```python
from build123d import *

# Parameters (mm, degrees)
F0_R        = 8.5
F0_R_2      = 7.5
F2_FACE_R   = 8.5
F2_FACE_R_2 = 7.5
F0_R_3      = 10
F6_R        = 10
F9_R        = 7.5
F14_R       = 8.5
F14_R_2     = 7.5
F12_R       = 7.5


with BuildPart() as f2:
    # F2: sweep along a path in F1
    with BuildLine(Plane.YZ) as f2_path:
        Line((0, 0), (0, 30))
    # F0 (on Top) → F2 (sweep)
    with BuildSketch(Plane.XY):
        Circle(F0_R)
        Circle(F0_R_2, mode=Mode.SUBTRACT)
    sweep(path=f2_path.line)

    # F4: sweep along a path in F1
    with BuildLine(Plane.YZ) as f4_path:
        Line((0, 30), (0, 0))
        Line((0, 0), (0, -30))
    # F2_face (on face) → F4 (sweep)
    with BuildSketch(Plane(origin=(0, 0, 0), x_dir=(1, 0, 0), z_dir=(0, 0, -1))):
        Circle(F2_FACE_R)
        Circle(F2_FACE_R_2, mode=Mode.SUBTRACT)
    sweep(path=f4_path.line)

    # F5: sweep along a path in F3
    with BuildLine(Plane.XZ) as f5_path:
        Line((0, 20), (0, 0))
        Line((0, 0), (0, -20))
    # F0 (on Top) → F5 (sweep)
    with BuildSketch(Plane.XY):
        Circle(F0_R_3)
        Circle(F0_R, mode=Mode.SUBTRACT)
    sweep(path=f5_path.line)

    # F8: sweep along a path in F7
    with BuildLine(Plane.YZ) as f8_path:
        Line((0, 0), (-30, 0))
    # F6 (on Front) → F8 (sweep, cut)
    with BuildSketch(Plane.XZ):
        Circle(F6_R)
    sweep(path=f8_path.line, mode=Mode.SUBTRACT)

    # F10: sweep along a path in F7
    with BuildLine(Plane.YZ) as f10_path:
        Line((0, 0), (-30, 0))
    # F6 (on Front) → F10 (sweep)
    with BuildSketch(Plane.XZ):
        Circle(F6_R)
    sweep(path=f10_path.line)

    # F11: sweep along a path in F7
    with BuildLine(Plane.YZ) as f11_path:
        Line((0, 0), (-30, 0))
    # F9 (on face) → F11 (sweep, cut)
    with BuildSketch(Plane.XZ):
        Circle(F9_R)
    sweep(path=f11_path.line, mode=Mode.SUBTRACT)

    # F15: sweep along a path in F13
    with BuildLine(Plane.XY) as f15_path:
        Line((0, -30), (0, -20))
    # F14 (on face) → F15 (sweep, cut)
    with BuildSketch(Plane.XZ.offset(30)):
        Circle(F14_R)
        Circle(F14_R_2, mode=Mode.SUBTRACT)
    sweep(path=f15_path.line, mode=Mode.SUBTRACT)

    # F16: sweep along a path in F3
    with BuildLine(Plane.XZ) as f16_path:
        Line((0, 20), (0, 0))
        Line((0, 0), (0, -20))
    # F12 (on Top) → F16 (sweep, cut)
    with BuildSketch(Plane.XY):
        Circle(F12_R)
    sweep(path=f16_path.line, mode=Mode.SUBTRACT)

    # F17: sweep along a path in F1
    with BuildLine(Plane.YZ) as f17_path:
        Line((0, 30), (0, 0))
        Line((0, 0), (0, -30))
    # F12 (on Top) → F17 (sweep, cut)
    with BuildSketch(Plane.XY):
        Circle(F12_R)
    sweep(path=f17_path.line, mode=Mode.SUBTRACT)


solid = f2.part
```
For this review, take the finished solid that the model builds, in its own axes (mm). A direction names the side the tool comes from. Round coordinates to 2 decimals unless told otherwise and drop trailing zeros. Order: outer loops, then holes, each group sorted by start corner. A loop starts at its lowest first (then second) coordinate and runs counter-clockwise, first axis right, second up. Notation, with made-up numbers: (68.5, -10.5) -> (96.5, -10.5) arc R13 ccw to (96.5, 4.5) -> close; hole circle Ø6 at (26.5, 16). An arc over 180 degrees is marked (long way). Use a Markdown table: item, result.
Item 1: Draft analysis for pull direction Z (two halves, no side actions). For faces 5 (the flat face through (-8, -20, 0)), 6 (the flat face through (-7.4, -30, 4.5)), 7 (the flat face through (0, -8, 30)), state which applies: +Z half, -Z half, draft (parallel to the pull), parting line (faces both ways), or undercut.
Resolved:
| item | result |
|---|---|
| face 5 | undercut |
| face 6 | draft |
| face 7 | +Z half |
Item 2: Machinability: for faces 1 (the cylindrical face through (-1.302, -18.543, 9.915)), 2 (the cylindrical face through (4.614, 8.872, -0.28)), 3 (the flat face through (-4.5, -7.4, -20)), 4 (the cylindrical face through (4.57, 7.167, 25.07)), which of the approach directions +Z, -Z, +X, -X, +Y, -Y give a long, thin tool a straight path to every point of the face, cutting with its end or side? Answer none if there is none.
Resolved:
| item | result |
|---|---|
| face 1 | -Y |
| face 2 | none |
| face 3 | -Z |
| face 4 | +Z |
Item 3: For pin 1 (1.5 mm diameter, centred on x = -5.5, z = 3.5, fed in from -Y); pin 2 (1.5 mm diameter, centred on x = 7, y = -9, fed in from -Z); pin 3 (12 mm diameter, centred on x = 0, z = 0, fed in from -Y), all flat-tipped, find the tip position at first contact; note any pin that passes through.
Resolved:
| item | result |
|---|---|
| pin 1 | stops at y = 4.15 |
| pin 2 | stops at z = -7.81 |
| pin 3 | stops at y = 4.5 |
Item 4: Take a section at C-C (z = 0). State the section outline as (x, y) points, plus the area to 3 significant figures.
Resolved:
| item | result |
|---|---|
| outline | (-10, -30) -> (-8.5, -30) -> (-8.5, -20) -> (-7.5, -20) -> (-7.5, 0) arc R7.5 cw to (7.5, 0) -> (7.5, -20) -> (8.5, -20) -> (8.5, -30) -> (10, -30) -> (10, 0) arc R10 ccw to (-10, 0) -> close |
| area | 199 mm² |
Item 5: Take a section at B-B (y = 4). State the section outline as (x, z) points, plus the area to 3 significant figures.
Resolved:
| item | result |
|---|---|
| outline | (-9.17, -20) -> (-7.5, -20) -> (-7.5, -30) -> (-6.34, -30) -> (-6.34, 30) -> (-7.5, 30) -> (-7.5, 20) -> (-9.17, 20) -> close; (6.34, -30) -> (7.5, -30) -> (7.5, -20) -> (9.17, -20) -> (9.17, 20) -> (7.5, 20) -> (7.5, 30) -> (6.34, 30) -> close |
| area | 272 mm² |
Item 6: Take a section at D-D (z = 21). State the section outline as (x, y) points.
Resolved:
| item | result |
|---|---|
| outline | circle Ø17 at (0, 0); hole circle Ø15 at (0, 0) |
Item 7: For line 1 along Z through (x, y) = (0, -26.75); line 2 along X through (y, z) = (0, 4), list the stretches that pass through material, from the lowest coordinate up. Write a range as [from, to].
Resolved:
| item | result |
|---|---|
| line 1 | z = [-10, -8.5], [8.5, 10] |
| line 2 | x = [-10, -7.5], [7.5, 10] |
Item 8: Take a section at A-A (x = 0). State the section outline as (y, z) points, plus the area to 4 significant figures.
Resolved:
| item | result |
|---|---|
| outline | (-30, -10) -> (-10, -10) -> (-10, -20) -> (-8.5, -20) -> (-8.5, -30) -> (-7.5, -30) -> (-7.5, -7.5) -> (-20, -7.5) -> (-20, -8.5) -> (-30, -8.5) -> close; (-30, 8.5) -> (-20, 8.5) -> (-20, 7.5) -> (-7.5, 7.5) -> (-7.5, 30) -> (-8.5, 30) -> (-8.5, 20) -> (-10, 20) -> (-10, 10) -> (-30, 10) -> close; (7.5, -30) -> (8.5, -30) -> (8.5, -20) -> (10, -20) -> (10, 20) -> (8.5, 20) -> (8.5, 30) -> (7.5, 30) -> close |
| area | 282.5 mm² |
